Can you work these out from the model? Positions are in its coordinate system, mm. A direction names the side the tool comes from. Give positions to 0.01 mm unless a question says otherwise; leave off trailing zeros. Order: outer loops, then holes, each group sorted by start corner. A loop starts at its lowest first (then second) coordinate and runs counter-clockwise, first axis right, second up.
Item 1: If I drill on line 1 along X through (y, z) = (0.85, 0); line 2 along X through (y, z) = (4.05, 0); line 3 along Z through (x, y) = (-0.25, 0.75), over which ranges is the centre line in solid material (lowest first)?
Item 2: I want a section at A-A, the plane z = 0. Write out the boundary of the cut face in (x, y).
Item 3: I want a section at B-B, the plane x = 7.5. Write out the boundary of the cut face in (y, z), then the cut area to 3 significant figures.
Item 4: I want a section at D-D, the plane x = 0. Write out the boundary of the cut face in (y, z).
Item 5: I'm going to push flat-ended pins straight in: pin 1 Ø5 at (x, z) = (7.5, 0) entering from -Y; pin 2 Ø2.5 at (x, z) = (1.5, -1.5) entering from +Y; pin 3 Ø6 at (y, z) = (-6.5, 0) entering from -X; pin 4 Ø12.5 at (x, z) = (-4, -6) entering from -Y. Where does each tip first touch, or does it pass through?
Item 6: I want a section at C-C, the plane z = -7.5. Write out the boundary of the cut face in (x, y).
Item 7: Which directions (+Z, -Z, +X, -X, +Y, -Y) give clear straight access to the entire face, cutting with the end or side of a thin tool? Please do faces 1 (the cylindrical face through (-3.905, 0.493, -0.867)), 2 (the cylindrical face through (1.352, -0.507, 4.292)), 3 (the flat face through (-5, 5, 0)).
```python
from build123d import *

# Parameters (mm, degrees)
SKETCH1_R                = 12.5
SKETCH1_R_2              = 4.5
SKETCH1_R_3              = 1.5
BOSS_EXTRUDE1_DEPTH      = 5
SKETCH1_3_R              = 4
BOSS_EXTRUDE2_DEPTH      = 13
BOSS_EXTRUDE3_DEPTH      = 1
BOSS_EXTRUDE3_DEPTH_BACK = 1
SKETCH1_4_R              = 4.5
SKETCH1_4_R_2            = 4


with BuildPart() as part:
    # Sketch1 → Boss-Extrude1 (new body)
    with BuildSketch(Plane(origin=(0, 0, 0), x_dir=(1, 0, 0), z_dir=(0, 1, 0))):
        with Locations(Location((0, 0, 0), (0, 0, 270))):
            Circle(SKETCH1_R)
        with Locations(Location((0, 0, 0), (0, 0, 270))):
            Circle(SKETCH1_R_2, mode=Mode.SUBTRACT)
        with Locations(Location((0, 7.5, 0), (0, 0, 270))):
            Circle(SKETCH1_R_3, mode=Mode.SUBTRACT)
        with Locations(Location((7.5, 0, 0), (0, 0, 270))):
            Circle(SKETCH1_R_3, mode=Mode.SUBTRACT)
        with Locations(Location((0, -7.5, 0), (0, 0, 270))):
            Circle(SKETCH1_R_3, mode=Mode.SUBTRACT)
        with Locations(Location((-7.5, 0, 0), (0, 0, 270))):
            Circle(SKETCH1_R_3, mode=Mode.SUBTRACT)
    extrude(amount=BOSS_EXTRUDE1_DEPTH)



with BuildPart() as body_2:
    # Sketch1_3 → Boss-Extrude2 (new body)
    with BuildSketch(Plane(origin=(0, 0, 0), x_dir=(1, 0, 0), z_dir=(0, 1, 0))):
        with Locations(Location((0, 0, 0), (0, 0, 270))):
            Circle(SKETCH1_3_R)
    extrude(amount=-BOSS_EXTRUDE2_DEPTH)


with BuildPart() as part_1:
    add(part.part)

    add(body_2.part)  # Boss-Extrude3 merges body 2
    # Sketch1_4 → Boss-Extrude3 (add, two sides: drawn at the far end of the back side and taken through both)
    with BuildSketch(Plane(origin=(0, 0, 0), x_dir=(1, 0, 0), z_dir=(0, 1, 0)).offset(-BOSS_EXTRUDE3_DEPTH_BACK)):
        with Locations(Location((0, 0, 0), (0, 0, 270))):
            Circle(SKETCH1_4_R)
        with Locations(Location((0, 0, 0), (0, 0, 270))):
            Circle(SKETCH1_4_R_2, mode=Mode.SUBTRACT)
    extrude(amount=BOSS_EXTRUDE3_DEPTH + BOSS_EXTRUDE3_DEPTH_BACK)


solid = part_1.part
```
Results list:
1. line 1: x = -12.5 to -9, -6 to -4, 4 to 6, 9 to 12.5
1. line 2: x = -12.5 to -9, -6 to -4.5, 4.5 to 6, 9 to 12.5
1. line 3: z = -12.5 to -8.98, -6.02 to -3.99, 3.99 to 6.02, 8.98 to 12.5
2. outline: (-12.5, 0) - (-9, 0) - (-9, 5) - (-12.5, 5) - close; (-6, 0) - (-4.5, 0) - (-4.5, -1) - (-4, -1) - (-4, -13) - (4, -13) - (4, -1) - (4.5, -1) - (4.5, 0) - (6, 0) - (6, 5) - (4.5, 5) - (4.5, 1) - (4, 1) - (4, 0) - (-4, 0) - (-4, 1) - (-4.5, 1) - (-4.5, 5) - (-6, 5) - close; (9, 0) - (12.5, 0) - (12.5, 5) - (9, 5) - close
3. outline: (0, -10) - (5, -10) - (5, -1.5) - (0, -1.5) - close; (0, 1.5) - (5, 1.5) - (5, 10) - (0, 10) - close
3. area: 85.0 mm2
4. outline: (-13, -4) - (-1, -4) - (-1, -4.5) - (0, -4.5) - (0, -6) - (5, -6) - (5, -4.5) - (1, -4.5) - (1, -4) - (0, -4) - (0, 4) - (1, 4) - (1, 4.5) - (5, 4.5) - (5, 6) - (0, 6) - (0, 4.5) - (-1, 4.5) - (-1, 4) - (-13, 4) - close; (0, -12.5) - (5, -12.5) - (5, -9) - (0, -9) - close; (0, 9) - (5, 9) - (5, 12.5) - (0, 12.5) - close
5. pin 1: stops at y = 0
5. pin 2: stops at y = 0
5. pin 3: stops at x = -4
5. pin 4: stops at y = -13
6. outline: (-10, 0) - (-1.5, 0) - (-1.5, 5) - (-10, 5) - close; (1.5, 0) - (10, 0) - (10, 5) - (1.5, 5) - close
7. face 1: +Y
7. face 2: -Y
7. face 3: +Z, -Z, +X, -X, +Y
